```python
from build123d import *

# Parameters (mm, degrees)
SKETCH1_W           = 35
SKETCH1_H           = 35
SKETCH1_R           = 4.6
SKETCH1_R_2         = 2
SKETCH1_R_3         = 2.5
BOSS_EXTRUDE1_DEPTH = 10


with BuildPart() as part:
    # Sketch1 → Boss-Extrude1 (new body)
    with BuildSketch(Plane.XY):
        with Locations((8.031937938, -5.058807352)):
            Rectangle(SKETCH1_W, SKETCH1_H)
        with Locations((8.031937938, -5.058807352)):
            Circle(SKETCH1_R, mode=Mode.SUBTRACT)
        with Locations((21.996404032, -19.023273446)):
            Circle(SKETCH1_R_2, mode=Mode.SUBTRACT)
        with Locations(Location((21.996404032, 8.905658742, 0), (0, 0, 180))):
            Circle(SKETCH1_R_2, mode=Mode.SUBTRACT)
        with Locations(Location((-5.932528156, -19.023273446, 0), (0, 0, 180))):
            Circle(SKETCH1_R_2, mode=Mode.SUBTRACT)
        with Locations((-5.932528156, 8.905658742)):
            Circle(SKETCH1_R_2, mode=Mode.SUBTRACT)
        with Locations((-4.468062062, -5.058807352)):
            Circle(SKETCH1_R_3, mode=Mode.SUBTRACT)
        with Locations(Location((20.531937938, -5.058807352, 0), (0, 0, 180))):
            Circle(SKETCH1_R_3, mode=Mode.SUBTRACT)
    extrude(amount=BOSS_EXTRUDE1_DEPTH)


solid = part.part
```
Part model, mm, in its own coordinate system. Coordinates: 2 decimals unless noted, no trailing zeros. Order: outer loops, then holes, each group sorted by start corner. A loop starts at its lowest first (then second) coordinate and runs counter-clockwise, first axis right, second up. Notation, with made-up numbers: (84.5, 40.5) - (91.5, 40.5) arc R12 ccw to (91.5, 58.5) - close; hole circle Ø5 at (1, 87). An arc over 180 degrees is marked (long way). Return JSON: item names as keys, results as strings. Group by question number.
Item 1: Cut at A-A (x = 19). List the corners of the cut face in (y, z).
Item 2: Drill centre lines: probe 1 along X at (y, z) = (-7, 3); probe 2 along Y at (x, z) = (20.5, 6); probe 3 along Y at (x, z) = (7.5, 4.5). Where is each one in solid material? Low to high. Write a range as from..to.
Item 3: Pull direction Y, two halves, no side cores. Call faces 1 (the face through (22.52, -3.54, 4.93)), 2 (the face through (25.532, -5, 5)), 3 (the face through (8, 12.441, 5)): pulls with the +Y half, pulls with the -Y half, needs draft (parallel to the pull), parting line crosses it, or undercut.
Item 4: Cut at B-B (z = 1.5). List the corners of the cut face in (x, y).
Item 5: Cut at D-D (x = 5.5). List the corners of the cut face in (y, z).
Item 6: Pin check, flat tip, straight feed: pin 1 (3 mm diameter, centred on x = -5.93, y = -19.02, fed in from -Z). Stop position of the tip, or through.
Item 7: Cut at C-C (x = -5.5). List the corners of the cut face in (y, z).
Check values:
{
 "1": {"outline": "(-22.56, 0) - (-7.03, 0) - (-7.03, 10) - (-22.56, 10) - close; (-3.08, 0) - (12.44, 0) - (12.44, 10) - (-3.08, 10) - close"},
 "2": {"probe 1": "x = -9.47..-6.04, -2.89..3.86, 12.2..18.96, 22.11..25.53", "probe 2": "y = -22.56..-20.35, -17.7..-7.56, -2.56..7.58, 10.23..12.44", "probe 3": "y = -22.56..-9.63, -0.49..12.44"},
 "3": {"face 1": "undercut", "face 2": "needs draft", "face 3": "pulls with the +Y half"},
 "4": {"outline": "(-9.47, -22.56) - (25.53, -22.56) - (25.53, 12.44) - (-9.47, 12.44) - close; hole circle Ø4 at (-5.93, -19.02); hole circle Ø4 at (-5.93, 8.91); hole circle Ø5 at (-4.47, -5.06); hole circle Ø9.2 at (8.03, -5.06); hole circle Ø5 at (20.53, -5.06); hole circle Ø4 at (22, -19.02); hole circle Ø4 at (22, 8.91)"},
 "5": {"outline": "(-22.56, 0) - (-8.9, 0) - (-8.9, 10) - (-22.56, 10) - close; (-1.22, 0) - (12.44, 0) - (12.44, 10) - (-1.22, 10) - close"},
 "6": {"pin 1": "passes through"},
 "7": {"outline": "(-22.56, 0) - (-20.98, 0) - (-20.98, 10) - (-22.56, 10) - close; (-17.07, 0) - (-7.34, 0) - (-7.34, 10) - (-17.07, 10) - close; (-2.78, 0) - (6.95, 0) - (6.95, 10) - (-2.78, 10) - close; (10.86, 0) - (12.44, 0) - (12.44, 10) - (10.86, 10) - close"}
}
